The figure shows three views and two pictorial views of one solid part (mm, origin at its lowest corner). Answer the questions. Give positions to 0.01 mm unless a question says otherwise; leave off trailing zeros. Loops run counter-clockwise (first coordinate to the right, second up) from the corner with the lowest first, then second, coordinate; pieces in that order, holes last. Notation, with made-up numbers: (73.5, 11.5) - (114.5, 11.5) arc R20 ccw to (114.5, 40.5) - close; hole circle Ø1 at (-39.5, 84). An arc over 180 degrees is marked (long way). One line per question, with ' | ' between items.
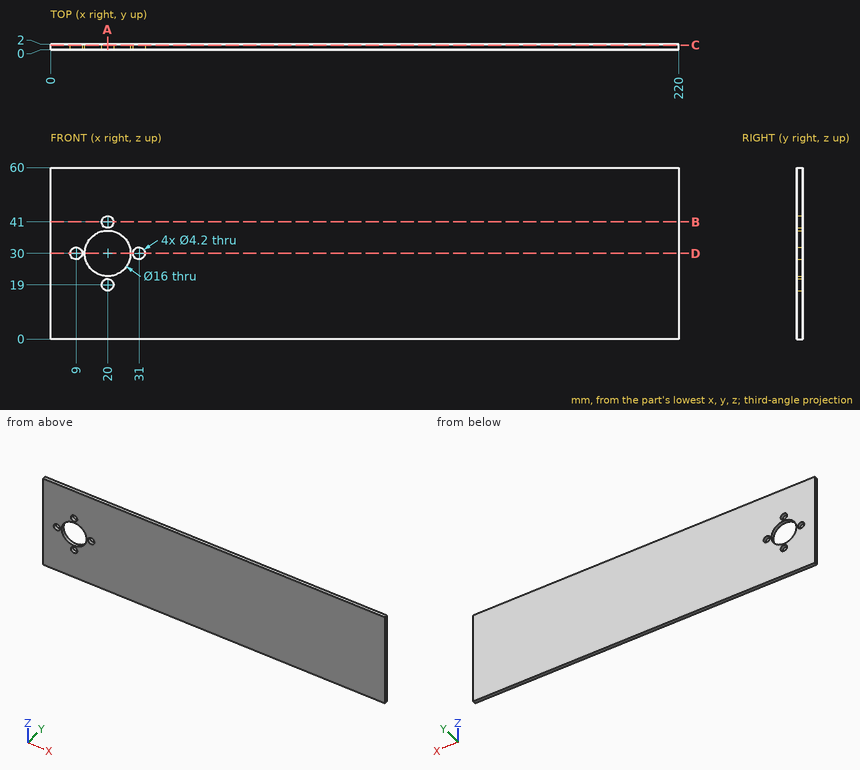
1. Find section B-B on z = 41. Write down the section's boundary in (x, y), then the cut area to 3 significant figures.
Evaluation:
outline: (0, 0) - (17.9, 0) - (17.9, 2) - (0, 2) - close; (22.1, 0) - (220, 0) - (220, 2) - (22.1, 2) - close | area: 432 mm2
2. Flat-ended cylindrical pins translate along their axes: pin 1 (8 mm diameter, centred on x = 165, z = 43, fed in from -Y); pin 2 (13 mm diameter, centred on x = 20, z = 30, fed in from -Y) (3 decimals). Find the tip coordinate at first contact, or state that the pin passes through.
Evaluation:
pin 1: y = 0 | pin 2: through
3. Find section D-D on z = 30. Write down the section's boundary in (x, y).
Evaluation:
outline: (0, 0) - (6.9, 0) - (6.9, 2) - (0, 2) - close; (11.1, 0) - (12, 0) - (12, 2) - (11.1, 2) - close; (28, 0) - (28.9, 0) - (28.9, 2) - (28, 2) - close; (33.1, 0) - (220, 0) - (220, 2) - (33.1, 2) - close
4. Consider L1, parallel to X at y = 1.3, z = 30; L2, parallel to Z at x = 20, y = 1.2; L3, parallel to Z at x = 21, y = 1.4. Determine where each line is inside the solid, lowest interval first.
Evaluation:
L1: 0 to 6.9, 11.1 to 12, 28 to 28.9, 33.1 to 220 | L2: 0 to 16.9, 21.1 to 22, 38 to 38.9, 43.1 to 60 | L3: 0 to 17.15, 20.85 to 22.06, 37.94 to 39.15, 42.85 to 60
5. Find section C-C on y = 1.6. Write down the section's boundary in (x, z), then the cut area to 3 significant figures.
Evaluation:
outline: (0, 0) - (220, 0) - (220, 60) - (0, 60) - close; hole circle Ø4.2 at (9, 30); hole circle Ø16 at (20, 30); hole circle Ø4.2 at (20, 19); hole circle Ø4.2 at (20, 41); hole circle Ø4.2 at (31, 30) | area: 12,900 mm2
6. Find section A-A on x = 20. Write down the section's boundary in (y, z).
Evaluation:
outline: (0, 0) - (2, 0) - (2, 16.9) - (0, 16.9) - close; (0, 21.1) - (2, 21.1) - (2, 22) - (0, 22) - close; (0, 38) - (2, 38) - (2, 38.9) - (0, 38.9) - close; (0, 43.1) - (2, 43.1) - (2, 60) - (0, 60) - close
